from build123d import *

# Parameters (mm, degrees)
SKETCH1_R           = 1.6
SKETCH1_W           = 70.2081528
SKETCH1_H           = 26
BOSS_EXTRUDE1_DEPTH = 1.5
SKETCH2_R           = 1.6
BOSS_EXTRUDE2_DEPTH = 1.5
CUT_EXTRUDE1_DEPTH  = 1.5


with BuildPart() as part:
    # Sketch1 → Boss-Extrude1 (new body)
    with BuildSketch(Plane.XY):
        with BuildLine():
            Line((0, -3), (20, -3))
            ThreePointArc((20, -3), (23, 0), (20, 3))
            Line((20, 3), (3, 3))
            Line((3, 3), (3, 13))
            Line((3, 13), (3, 29))
            Line((3, 29), (20, 29))
            ThreePointArc((20, 29), (23, 32), (20, 35))
            Line((20, 35), (0, 35))
            Line((0, 35), (-76.2081528, 35))
            Line((-76.2081528, 35), (-96.2081528, 35))
            ThreePointArc((-96.2081528, 35), (-99.2081528, 32), (-96.2081528, 29))
            Line((-96.2081528, 29), (-79.2081528, 29))
            Line((-79.2081528, 29), (-79.2081528, 14.5))
            Line((-79.2081528, 14.5), (-79.2081528, 3))
            Line((-79.2081528, 3), (-96.2081528, 3))
            ThreePointArc((-96.2081528, 3), (-99.2081528, 0), (-96.2081528, -3))
            Line((-96.2081528, -3), (-76.2081528, -3))
            Line((-76.2081528, -3), (0, -3))
        make_face()
        with Locations((-76.2081528, 0)):
            Circle(SKETCH1_R, mode=Mode.SUBTRACT)
        with Locations((-76.2081528, 32)):
            Circle(SKETCH1_R, mode=Mode.SUBTRACT)
        Circle(SKETCH1_R, mode=Mode.SUBTRACT)
        with Locations((20, 0)):
            Circle(SKETCH1_R, mode=Mode.SUBTRACT)
        with Locations((0, 32)):
            Circle(SKETCH1_R, mode=Mode.SUBTRACT)
        with Locations((20, 32)):
            Circle(SKETCH1_R, mode=Mode.SUBTRACT)
        with Locations((-96.2081528, 32)):
            Circle(SKETCH1_R, mode=Mode.SUBTRACT)
        with Locations((-96.2081528, 0)):
            Circle(SKETCH1_R, mode=Mode.SUBTRACT)
        with Locations((-38.1040764, 16)):
            Rectangle(SKETCH1_W, SKETCH1_H, mode=Mode.SUBTRACT)
    extrude(amount=BOSS_EXTRUDE1_DEPTH)

    # Sketch2 → Boss-Extrude2 (add)
    with BuildSketch(Plane.XY.offset(1.5)):
        with BuildLine():
            Line((-74.086832456, 34.121320344), (-68.601551082, 28.636038969))
            Line((-68.601551082, 28.636038969), (-7.606601718, 28.636038969))
            Line((-7.606601718, 28.636038969), (-2.121320344, 34.121320344))
            ThreePointArc((-2.121320344, 34.121320344), (2.121320344, 34.121320344), (2.121320344, 29.878679656))
            Line((2.121320344, 29.878679656), (-4.242640687, 23.514718626))
            ThreePointArc((-4.242640687, 23.514718626), (-5.215910734, 22.864400372), (-6.363961031, 22.636038969))
            Line((-6.363961031, 22.636038969), (-69.844191769, 22.636038969))
            ThreePointArc((-69.844191769, 22.636038969), (-70.992242066, 22.864400372), (-71.965512113, 23.514718626))
            Line((-71.965512113, 23.514718626), (-78.329473144, 29.878679656))
            ThreePointArc((-78.329473144, 29.878679656), (-78.329473144, 34.121320344), (-74.086832456, 34.121320344))
        make_face()
        with Locations((0, 32)):
            Circle(SKETCH2_R, mode=Mode.SUBTRACT)
        with Locations((-76.2081528, 32)):
            Circle(SKETCH2_R, mode=Mode.SUBTRACT)
        with BuildLine():
            Line((-69.844191769, 9.363961031), (-6.363961031, 9.363961031))
            ThreePointArc((-6.363961031, 9.363961031), (-5.215910734, 9.135599628), (-4.242640687, 8.485281374))
            Line((-4.242640687, 8.485281374), (2.121320344, 2.121320344))
            ThreePointArc((2.121320344, 2.121320344), (2.121320344, -2.121320344), (-2.121320344, -2.121320344))
            Line((-2.121320344, -2.121320344), (-7.606601718, 3.363961031))
            Line((-7.606601718, 3.363961031), (-68.601551082, 3.363961031))
            Line((-68.601551082, 3.363961031), (-74.086832456, -2.121320344))
            ThreePointArc((-74.086832456, -2.121320344), (-78.329473144, -2.121320344), (-78.329473144, 2.121320344))
            Line((-78.329473144, 2.121320344), (-71.965512113, 8.485281374))
            ThreePointArc((-71.965512113, 8.485281374), (-70.992242066, 9.135599628), (-69.844191769, 9.363961031))
        make_face()
        with Locations((-76.2081528, 0)):
            Circle(SKETCH2_R, mode=Mode.SUBTRACT)
        Circle(SKETCH2_R, mode=Mode.SUBTRACT)
    extrude(amount=-BOSS_EXTRUDE2_DEPTH)

    # Sketch3 → Cut-Extrude1 (cut)
    with BuildSketch(Plane.XY.offset(1.5)):
        with BuildLine():
            Line((-68.601551082, 28.636038969), (-74.088420945, 34.12061745))
            ThreePointArc((-74.088420945, 34.12061745), (-75.061011799, 34.770261546), (-76.2081528, 34.998379814))
            Line((-76.2081528, 34.998379814), (-76.2081528, 40.296736943))
            Line((-76.2081528, 40.296736943), (0, 40.296736943))
            Line((0, 40.296736943), (0, 35.000078273))
            ThreePointArc((0, 35.000078273), (-1.148094234, 34.77170512), (-2.121397096, 34.121354286))
            Line((-2.121397096, 34.121354286), (-7.606601718, 28.636038969))
            Line((-7.606601718, 28.636038969), (-68.601551082, 28.636038969))
        make_face()
        with BuildLine():
            Line((-76.2081528, -8.296736943), (-76.2081528, -2.998379814))
            ThreePointArc((-76.2081528, -2.998379814), (-75.061011799, -2.770261546), (-74.088420945, -2.12061745))
            Line((-74.088420945, -2.12061745), (-68.601551082, 3.363961031))
            Line((-68.601551082, 3.363961031), (-7.606601718, 3.363961031))
            Line((-7.606601718, 3.363961031), (-2.121397096, -2.121354286))
            ThreePointArc((-2.121397096, -2.121354286), (-1.148094234, -2.77170512), (0, -3.000078273))
            Line((0, -3.000078273), (0, -8.296736943))
            Line((0, -8.296736943), (-76.2081528, -8.296736943))
        make_face()
    extrude(amount=-CUT_EXTRUDE1_DEPTH, mode=Mode.SUBTRACT)


solid = part.part
Input: part model. Units: mm. Frame: model coordinates. A direction names the side the tool comes from. Coordinates: 2 decimals unless noted, no trailing zeros. Order: outer loops, then holes, each group sorted by start corner. A loop starts at its lowest first (then second) coordinate and runs counter-clockwise, first axis right, second up. Notation, with made-up numbers: M 12.5,71.25 L 56.5,71.25 A18 cw 56.5,94.25 Z; hole C 58.5,76.5 d3. An arc over 180 degrees is marked long. One line per question, with ' | ' between items.
Item 1: Section C-C (y = 0). Output: boundary loops of the cut face in (x, z).
Geometry results:
outline: M -99.21,0 L -97.81,0 L -97.81,1.5 L -99.21,1.5 Z; M -94.61,0 L -77.81,0 L -77.81,1.5 L -94.61,1.5 Z; M -74.61,0 L -71.97,0 L -71.97,1.5 L -74.61,1.5 Z; M -4.24,0 L -1.6,0 L -1.6,1.5 L -4.24,1.5 Z; M 1.6,0 L 18.4,0 L 18.4,1.5 L 1.6,1.5 Z; M 21.6,0 L 23,0 L 23,1.5 L 21.6,1.5 Z
Item 2: Pin query (flat end, axial travel): pin 1 (2.5 mm diameter, centred on x = -96.21, y = 0, fed in from -Z); pin 2 (0.8 mm diameter, centred on y = 17, z = 0.5, fed in from +X). Return the tip coordinate at first contact, or that it passes through.
Geometry results:
pin 1: passes through | pin 2: stops at x = 3
Item 3: Reachability of faces 1 (the flat face through (-71.383, 0.583, 0.76)), 2 (the cylindrical face through (23, 32, 1)), 3 (the flat face through (-4.646, 31.597, 0.76)) from +Z, -Z, +X, -X, +Y, -Y: full face, straight path, thin tool, end or side. Return the list, or none.
Geometry results:
face 1: +Z, -Z, -Y | face 2: +Z, -Z, +X | face 3: +Z, -Z, +Y
Item 4: Ray query, line 1 along Y through (x, z) = (0, 0.4); line 2 along Y through (x, z) = (-27, 0.95); line 3 along Y through (x, z) = (11.5, 1.1). Return the intervals inside material, ascending.
Geometry results:
line 1: y = -3 to -1.6, 1.6 to 30.4, 33.6 to 35 | line 2: y = 3.36 to 9.36, 22.64 to 28.64 | line 3: y = -3 to 3, 29 to 35
Item 5: Draft query along X for faces 4 (the cylindrical face through (-99.207, 0.066, 0.74)), 5 (the cylindrical face through (18.73, 31.03, 0.74)), 6 (the cylindrical face through (-1.27, -0.97, 0.74)), 7 (the flat face through (-25, 8, 1.5)). Return one class per face: released by +X, released by -X, zero draft, split by the parting line, or undercut.
Geometry results:
face 4: released by -X | face 5: undercut | face 6: undercut | face 7: zero draft
Item 6: Section D-D (y = 26). Output: boundary loops of the cut face in (x, z), then the cut area to 3 significant figures.
Geometry results:
outline: M -79.21,0 L 3,0 L 3,1.5 L -79.21,1.5 Z | area: 123 mm^2
Item 7: Section B-B (x = 12). Output: boundary loops of the cut face in (y, z), then the cut area to 3 significant figures.
Geometry results:
outline: M -3,0 L 3,0 L 3,1.5 L -3,1.5 Z; M 29,0 L 35,0 L 35,1.5 L 29,1.5 Z | area: 18.0 mm^2
Item 8: Section A-A (y = 14). Output: boundary loops of the cut face in (x, z), then the cut area to 3 significant figures.
Geometry results:
outline: M -79.21,0 L -73.21,0 L -73.21,1.5 L -79.21,1.5 Z; M -3,0 L 3,0 L 3,1.5 L -3,1.5 Z | area: 18.0 mm^2
